Check sheet for the modelled part. Datum: model origin and axes. Units: mm. A direction names the side the tool comes from. Give positions to 0.01 mm unless a question says otherwise; leave off trailing zeros. Write each loop counter-clockwise with the first axis right and the second up, starting at its lowest first coordinate (ties: lowest second). Pieces come first, ordered by that corner, then holes. Notation, with made-up numbers: (-21.5, -34) -> (4.5, -34) arc R19 ccw to (4.5, -3) -> close; hole circle Ø9 at (63.25, -25). An arc over 180 degrees is marked (long way). Use a Markdown table: item, result. Add a question column.
1. Gauge pin test, flat ends, axial feed: P1, Ø6.5, axis at x = -0.5, z = 264.5, coming from the +Y side; P2, Ø1, axis at x = 5, z = 68.5, coming from the +Y side; P3, Ø5, axis at x = -5, z = -60.5, coming from the +Y side; P4, Ø4.5, axis at x = 0.5, y = 5, coming from the -Z side. Record the tip position at first contact, or that the pin passes through.
2. Scan lines: probe 1 along Y at (x, z) = (0.75, 123.5); probe 2 along Z at (x, y) = (2.5, 3.5); probe 3 along Y at (x, z) = (-3, 150). Record each from-to range of solid material in increasing order. Write a range as [from, to].
3. Cross-section at B-B (x = 4). Enter the section's corners in (y, z), then the cut area to 3 significant figures.
4. Set-up check for faces 1 (the cylindrical face through (3.23, -6.21, 3.78)), 2 (the flat face through (0, 3, 263)), 3 (the flat face through (0, 3, -263)): record each of +Z, -Z, +X, -X, +Y, -Y from which the full face is reachable in a straight line by a thin tool's end or side.
5. Cross-section at A-A (z = -53.5). Enter the section's corners in (x, y), then the cut area to 3 significant figures.
from build123d import *

# Parameters (mm, degrees)
SKETCH1_R           = 7
BOSS_EXTRUDE1_DEPTH = 270
CUT_EXTRUDE1_DEPTH  = 15.1
CUT_EXTRUDE2_START  = -145
SKETCH3_W           = 3.175
SKETCH3_H           = 3.175
CUT_EXTRUDE2_DEPTH  = 75


with BuildPart() as part:
    # Sketch1 → Boss-Extrude1 (new, symmetric)
    with BuildSketch(Plane.XY):
        Circle(SKETCH1_R)
    extrude(amount=BOSS_EXTRUDE1_DEPTH, both=True)

    # Sketch2 → Cut-Extrude1 (cut)
    with BuildSketch(Plane.XY.offset(270)):
        with BuildLine():
            Line((-6.32455532, 3), (6.32455532, 3))
            ThreePointArc((6.32455532, 3), (0, 7), (-6.32455532, 3))
        make_face()
    cut_extrude1 = extrude(amount=-CUT_EXTRUDE1_DEPTH, mode=Mode.SUBTRACT)

    # Sketch3 → Cut-Extrude2 (cut)
    with BuildSketch(Plane.XY.offset(270).offset(CUT_EXTRUDE2_START)):
        with Locations((0, 7)):
            Rectangle(SKETCH3_W, SKETCH3_H)
    extrude(amount=-CUT_EXTRUDE2_DEPTH, mode=Mode.SUBTRACT)

    # Mirror1: Cut-Extrude1 across plane
    add(cut_extrude1.mirror(Plane.XY), mode=Mode.SUBTRACT)


solid = part.part
Worked answers:
| question | item | result |
|---|---|---|
| 1 | P1 | stops at y = 3 |
| 1 | P2 | stops at y = 5.36 |
| 1 | P3 | stops at y = 6.54 |
| 1 | P4 | stops at z = -270 |
| 2 | probe 1 | y = [-6.96, 5.41] |
| 2 | probe 2 | z = [-254.9, 254.9] |
| 2 | probe 3 | y = [-6.32, 6.32] |
| 3 | outline | (-5.74, -270) -> (3, -270) -> (3, -254.9) -> (5.74, -254.9) -> (5.74, 254.9) -> (3, 254.9) -> (3, 270) -> (-5.74, 270) -> close |
| 3 | area | 6,120 mm² |
| 4 | face 1 | +Z, -Z |
| 4 | face 2 | +Z, +X, -X, +Y |
| 4 | face 3 | -Z, +X, -X, +Y |
| 5 | outline | circle Ø14 at (0, 0) |
| 5 | area | 154 mm² |
